from build123d import *

# Parameters (mm, degrees)
BOSS_EXTRUDE1_DEPTH = 59
SKETCH2_R           = 5
CUT_EXTRUDE1_DEPTH  = 4


with BuildPart() as part:
    # Sketch1 → Boss-Extrude1 (new body)
    with BuildSketch(Plane(origin=(0, 0, 0), x_dir=(1, 0, 0), z_dir=(0, 1, 0))):
        with BuildLine():
            Line((-18.608695652, -27.695652174), (17.391304348, -27.695652174))
            ThreePointArc((17.391304348, -27.695652174), (18.80551791, -27.109865736), (19.391304348, -25.695652174))
            Line((19.391304348, -25.695652174), (19.391304348, 10.304347826))
            ThreePointArc((19.391304348, 10.304347826), (18.80551791, 11.718561388), (17.391304348, 12.304347826))
            Line((17.391304348, 12.304347826), (-18.608695652, 12.304347826))
            ThreePointArc((-18.608695652, 12.304347826), (-20.022909215, 11.718561388), (-20.608695652, 10.304347826))
            Line((-20.608695652, 10.304347826), (-20.608695652, -25.695652174))
            ThreePointArc((-20.608695652, -25.695652174), (-20.022909215, -27.109865736), (-18.608695652, -27.695652174))
        make_face()
    extrude(amount=BOSS_EXTRUDE1_DEPTH)

    # Sketch2 → Cut-Extrude1 (cut)
    with BuildSketch(Plane.XZ):
        with Locations(Location((-0.608695652, 7.695652174, 0), (0, 0, 270))):
            Circle(SKETCH2_R)
    extrude(amount=-CUT_EXTRUDE1_DEPTH, mode=Mode.SUBTRACT)


solid = part.part
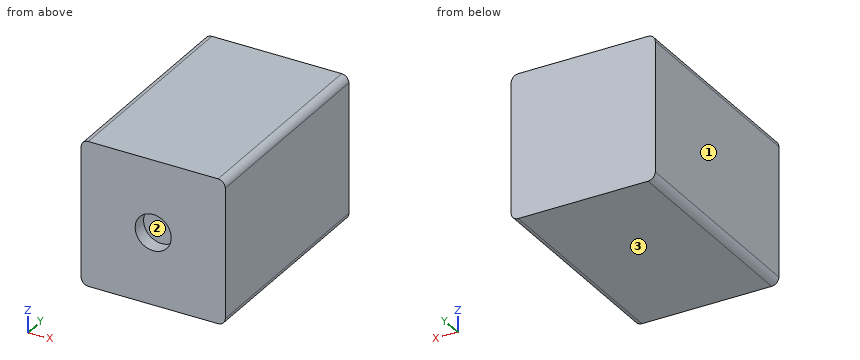
For this review, take the finished solid that the model builds, in its own axes (mm). Face numbers are marked on the shaded views. Round coordinates to 2 decimals unless told otherwise and drop trailing zeros. Order: outer loops, then holes, each group sorted by start corner. A loop starts at its lowest first (then second) coordinate and runs counter-clockwise, first axis right, second up. Notation, with made-up numbers: (-13, -27.75) -> (12, -27.75) arc R16 cw to (12, -12.75) -> close; hole circle Ø6 at (73, -8.75). An arc over 180 degrees is marked (long way). Write item = value, one per line. Start each with the question number.
1) To check wall thickness, follow line 1 (Y direction, x = -3, z = 8). State the ranges of the line that lie inside material, in increasing order. Write a range as from..to.
2) The part is to be moulded in two halves that separate along Z. For the marked faces 1, 2 and 3, say which applies: +Z half, -Z half, draft (parallel to the pull), parting line (faces both ways), or undercut.
3) Insertion check: pin 1 (3 mm diameter, centred on x = 0.5, z = 5.5, fed in from -Y). The pin has a flat end and moves straight along its axis. Give the tip position at first contact, or say it passes through.
4) Take a section at A-A on x = -1.5. State the section outline as (y, z) points.
Verdict:
q1.line_1 = 4..59
q2.face_1 = draft
q2.face_2 = undercut
q2.face_3 = -Z half
q3.pin_1 = 4
q4.outline = (0, -12.3) -> (59, -12.3) -> (59, 27.7) -> (0, 27.7) -> (0, 12.62) -> (4, 12.62) -> (4, 2.78) -> (0, 2.78) -> close
